Geometry: final body of the model. Coordinates: model frame, mm. Face numbers are marked on the shaded views. A direction names the side the tool comes from. Round coordinates to 2 decimals unless told otherwise and drop trailing zeros. Loops run counter-clockwise (first coordinate to the right, second up) from the corner with the lowest first, then second, coordinate; pieces in that order, holes last. Notation, with made-up numbers: (6.25, -24.5) - (51.25, -24.5) arc R25 ccw to (51.25, 12.5) - close; hole circle Ø11 at (-31, 60). An arc over 180 degrees is marked (long way). Use CSV: the item, a comma, the result in double quotes.
from build123d import *

# Parameters (mm, degrees)
ESQUISSE1_W             = 75
ESQUISSE1_H             = 50
BOSS_EXTRU_1_DEPTH      = 3
ESQUISSE2_W             = 3
ESQUISSE2_H             = 50
BOSS_EXTRU_2_DEPTH      = 47
ESQUISSE3_R             = 10.5
ESQUISSE3_R_2           = 1.5
ENL_V_MAT_EXTRU_1_DEPTH = 3
BOSS_EXTRU_3_DEPTH      = 3
BOSS_EXTRU_4_DEPTH      = 3
ESQUISSE6_R             = 1.5
ENL_V_MAT_EXTRU_2_DEPTH = 3


with BuildPart() as part:
    # Esquisse1 → Boss.-Extru.1 (new body)
    with BuildSketch(Plane(origin=(0, 0, 0), x_dir=(1, 0, 0), z_dir=(0, 1, 0))):
        with Locations((37.5, 25)):
            Rectangle(ESQUISSE1_W, ESQUISSE1_H)
    extrude(amount=BOSS_EXTRU_1_DEPTH)

    # Esquisse2 → Boss.-Extru.2 (add)
    with BuildSketch(Plane(origin=(0, 3, 0), x_dir=(1, 0, 0), z_dir=(0, 1, 0))):
        with Locations((1.5, 25)):
            Rectangle(ESQUISSE2_W, ESQUISSE2_H)
    extrude(amount=BOSS_EXTRU_2_DEPTH)

    # Esquisse3 → Enlèv. mat.-Extru.1 (cut)
    with BuildSketch(Plane.ZY):
        with Locations((-25, 28)):
            Circle(ESQUISSE3_R)
        with Locations((-12, 28)):
            Circle(ESQUISSE3_R_2)
        with Locations((-25, 15)):
            Circle(ESQUISSE3_R_2)
        with Locations((-38, 28)):
            Circle(ESQUISSE3_R_2)
        with Locations((-25, 41)):
            Circle(ESQUISSE3_R_2)
    extrude(amount=-ENL_V_MAT_EXTRU_1_DEPTH, mode=Mode.SUBTRACT)

    # Esquisse4 → Boss.-Extru.3 (add)
    with BuildSketch(Plane.XY):
        Polygon((3, 50), (75, 3), (3, 3), align=None)
    extrude(amount=-BOSS_EXTRU_3_DEPTH)

    # Esquisse5 → Boss.-Extru.4 (add)
    with BuildSketch(Plane(origin=(0, 0, -50), x_dir=(-1, 0, 0), z_dir=(0, 0, -1))):
        Polygon((-75, 3), (-3, 3), (-3, 50), align=None)
    extrude(amount=-BOSS_EXTRU_4_DEPTH)

    # Esquisse6 → Enlèv. mat.-Extru.2 (cut)
    with BuildSketch(Plane(origin=(0, 3, 0), x_dir=(1, 0, 0), z_dir=(0, 1, 0))):
        with Locations(Location((7, 43, 0), (0, 0, 270))):
            Circle(ESQUISSE6_R)
        with Locations(Location((68, 43, 0), (0, 0, 270))):
            Circle(ESQUISSE6_R)
        with Locations(Location((68, 7, 0), (0, 0, 270))):
            Circle(ESQUISSE6_R)
        with Locations(Location((7, 7, 0), (0, 0, 270))):
            Circle(ESQUISSE6_R)
    extrude(amount=-ENL_V_MAT_EXTRU_2_DEPTH, mode=Mode.SUBTRACT)


solid = part.part
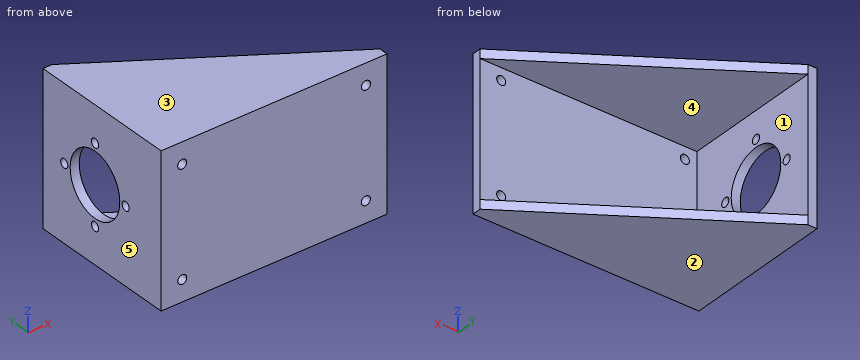
Item 1: Section D-D on x = 7. Return the cut outline in (y, z), plus the area to 3 significant figures.
Final values:
outline,"(0, -50) - (47.39, -50) - (47.39, -47) - (3, -47) - (3, -44.5) - (0, -44.5) - close; (0, -41.5) - (3, -41.5) - (3, -8.5) - (0, -8.5) - close; (0, -5.5) - (3, -5.5) - (3, -3) - (47.39, -3) - (47.39, 0) - (0, 0) - close"
area,"398 mm²"
Item 2: Section C-C on y = 21. Return the cut outline in (x, z), plus the area to 3 significant figures.
Final values:
outline,"(0, -50) - (47.43, -50) - (47.43, -47) - (3, -47) - (3, -32.83) - (0, -32.83) - close; (0, -17.17) - (3, -17.17) - (3, -3) - (47.43, -3) - (47.43, 0) - (0, 0) - close"
area,"370 mm²"
Item 3: Mould query, pull axis Z, two halves, no side actions, for the marked faces 1, 2 and 3. Classes: released by +Z, released by -Z, zero draft, split by the parting line, or undercut.
Final values:
face 1,"undercut"
face 2,"released by -Z"
face 3,"released by +Z"
Item 4: Material intervals for line 1 (Z direction, x = 68, y = 1.55); line 2 (X direction, y = 1, z = -43); line 3 (Z direction, x = 19, y = 10.5), sorted ascending.
Final values:
line 1,"z = -50 to -44.5, -41.5 to -8.5, -5.5 to 0"
line 2,"x = 0 to 5.5, 8.5 to 66.5, 69.5 to 75"
line 3,"z = -50 to -47, -3 to 0"
Item 5: Section A-A on z = -7. Return the cut outline in (x, y).
Final values:
outline,"(0, 0) - (5.5, 0) - (5.5, 3) - (3, 3) - (3, 50) - (0, 50) - close; (8.5, 0) - (66.5, 0) - (66.5, 3) - (8.5, 3) - close; (69.5, 0) - (75, 0) - (75, 3) - (69.5, 3) - close"
Item 6: Section B-B on z = -12. Return the cut outline in (x, y), plus the area to 3 significant figures.
Final values:
outline,"(0, 0) - (75, 0) - (75, 3) - (3, 3) - (3, 26.5) - (0, 26.5) - close; (0, 29.5) - (3, 29.5) - (3, 50) - (0, 50) - close"
area,"357 mm²"
Item 7: Reachability of the marked faces 4 and 5 from +Z, -Z, +X, -X, +Y, -Y: full face, straight path, thin tool, end or side. Return the list, or none.
Final values:
face 4,"+X, +Y"
face 5,"+Z, -Z, -X, +Y, -Y"
Item 8: Pin query (flat end, axial travel): P1, Ø6, axis at y = 44.5, z = -11.5, coming from the +X side; P2, Ø4, axis at x = 68, z = -43, coming from the +Y side; P3, Ø1.8, axis at x = 7, z = -7, coming from the +Y side. Return the tip coordinate at first contact, or that it passes through.
Final values:
P1,"stops at x = 3"
P2,"stops at y = 3"
P3,"passes through"
